Could you check a few things on this model? Use its own coordinates, in mm. Face numbers are marked on the shaded views. A direction names the side the tool comes from. Give positions to 0.01 mm unless a question says otherwise; leave off trailing zeros. Write each loop counter-clockwise with the first axis right and the second up, starting at its lowest first coordinate (ties: lowest second). Pieces come first, ordered by that corner, then holes. Notation, with made-up numbers: (67.25, -16.5) - (111.25, -16.5) arc R29 cw to (111.25, 10.5) - close; hole circle Ø2 at (-29.5, 24). An arc over 180 degrees is marked (long way). Answer as a JSON object with one key per item and string values. Group by question number.
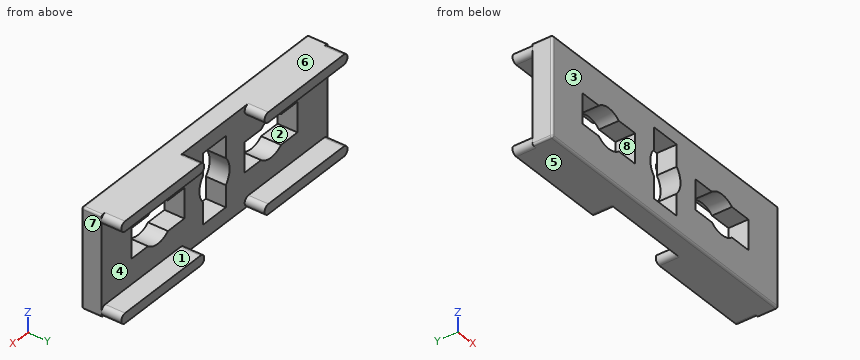
```python
from build123d import *

# Parameters (mm, degrees)
SKETCH_1_W            = 30
SKETCH_1_H            = 10
EXTRUDE_1_DEPTH       = 2
EXTRUDE_2_DEPTH       = 2
MIRROR_2_COPY_1_DEPTH = 2
CUT_EXTRUDE_1_REACH   = 17.937
CUT_EXTRUDE_2_REACH   = 17.937
FILLET_1_R            = 0.2


with BuildPart() as part:
    # 草图1 → 凸台-拉伸1 (new body)
    with BuildSketch(Plane(origin=(0, 0, 0), x_dir=(1, 0, 0), z_dir=(0, 1, 0))):
        Rectangle(SKETCH_1_W, SKETCH_1_H)
    extrude(amount=EXTRUDE_1_DEPTH)

    # 草图2 → 凸台-拉伸2 (add)
    with BuildSketch(Plane(origin=(0, 2, 0), x_dir=(1, 0, 0), z_dir=(0, 1, 0))):
        with BuildLine():
            Line((-14.5, 4), (-4.5, 4))
            ThreePointArc((-4.5, 4), (-4, 4.5), (-4.5, 5))
            Line((-4.5, 5), (-14.5, 5))
            ThreePointArc((-14.5, 5), (-15, 4.5), (-14.5, 4))
        make_face()
    extrude_2 = extrude(amount=EXTRUDE_2_DEPTH)

    # 镜向1: 凸台-拉伸2 across plane
    add(extrude_2.mirror(Plane.XY))

    # 镜向2: 凸台-拉伸2 across plane
    add(extrude_2.mirror(Plane(origin=(0, 0, 0), x_dir=(0, 0, 1), z_dir=(1, 0, 0))))

    # 镜向2 copy 1 sketch → 镜向2 copy 1 (add)
    with BuildSketch(Plane(origin=(0, 2, 0), x_dir=(-1, 0, 0), z_dir=(0, 1, 0))):
        with BuildLine():
            Line((-14.5, 4), (-4.5, 4))
            ThreePointArc((-4.5, 4), (-4, 4.5), (-4.5, 5))
            Line((-4.5, 5), (-14.5, 5))
            ThreePointArc((-14.5, 5), (-15, 4.5), (-14.5, 4))
        make_face()
    extrude(amount=MIRROR_2_COPY_1_DEPTH)

    # 草图3 → 切除-拉伸1 (cut, up to next)
    with BuildSketch(Plane(origin=(0, 2, 0), x_dir=(1, 0, 0), z_dir=(0, 1, 0)), mode=Mode.PRIVATE) as cut_extrude_1_sk1:
        with BuildLine():
            Line((1.5, -3.5), (-1.5, -3.5))
            Line((-1.5, -3.5), (-1.5, -1.322875656))
            ThreePointArc((-1.5, -1.322875656), (-2, 0), (-1.5, 1.322875656))
            Line((-1.5, 1.322875656), (-1.5, 3.5))
            Line((-1.5, 3.5), (1.5, 3.5))
            Line((1.5, 3.5), (1.5, 1.322875656))
            ThreePointArc((1.5, 1.322875656), (2, 0), (1.5, -1.322875656))
            Line((1.5, -1.322875656), (1.5, -3.5))
        make_face()
    cut_extrude_1_tool1 = extrude(cut_extrude_1_sk1.sketch, amount=-CUT_EXTRUDE_1_REACH, mode=Mode.PRIVATE) & part.part
    add(cut_extrude_1_tool1.solids().sort_by_distance((0, 2, 0))[0], mode=Mode.SUBTRACT)

    # 草图4 → 切除-拉伸2 (cut, up to next)
    with BuildSketch(Plane(origin=(0, 2, 0), x_dir=(1, 0, 0), z_dir=(0, 1, 0)), mode=Mode.PRIVATE) as cut_extrude_2_sk1:
        with BuildLine():
            Line((-4, 1.5), (-4, -1.5))
            Line((-4, -1.5), (-6.177124344, -1.5))
            ThreePointArc((-6.177124344, -1.5), (-7.5, -2), (-8.822875656, -1.5))
            Line((-8.822875656, -1.5), (-11, -1.5))
            Line((-11, -1.5), (-11, 1.5))
            Line((-11, 1.5), (-8.822875656, 1.5))
            ThreePointArc((-8.822875656, 1.5), (-7.5, 2), (-6.177124344, 1.5))
            Line((-6.177124344, 1.5), (-4, 1.5))
        make_face()
    cut_extrude_2_tool1 = extrude(cut_extrude_2_sk1.sketch, amount=-CUT_EXTRUDE_2_REACH, mode=Mode.PRIVATE) & part.part
    cut_extrude_2 = cut_extrude_2_tool1.solids().sort_by_distance((-7.5, 2, 0))[0]
    add(cut_extrude_2, mode=Mode.SUBTRACT)

    # 镜向3: 切除-拉伸2 across plane
    add(cut_extrude_2.mirror(Plane(origin=(0, 0, 0), x_dir=(0, 0, 1), z_dir=(1, 0, 0))), mode=Mode.SUBTRACT)

    # 圆角1
    fillet_1_edges = [part.edges().sort_by_distance(p)[0] for p in [
        (0, 0, 5),
        (-15, 1, 5),
        (-15, 0, 0),
        (-15, 1, -5),
        (0, 0, -5),
        (15, 0, 0),
        (15, 1, -5),
        (15, 1, 5),
    ]]
    fillet(fillet_1_edges, radius=FILLET_1_R)


solid = part.part
```
(1) I need wall thicknesses on L1, parallel to X at y = 1.05, z = 0; L2, parallel to Z at x = 9, y = 2.3; L3, parallel to X at y = 1.25, z = -0.5. Which ranges of each line are inside material? Lowest first, please.
(2) If we mould it in two halves opening along X, with no side actions, what happens to the marked faces 6, 7 and 8? For each: +X half, -X half, draft (parallel to the pull), parting line (faces both ways), or undercut.
(3) Will this pin go through, and if not, where does the flat tip stop? P1, Ø3, axis at x = 1, z = 0, coming from the +Y side.
(4) I want a section at A-A, the plane x = 5.25. Please give me the cut outline in (y, z).
(5) I want a section at B-B, the plane y = 2.65. Please give me the cut outline in (x, z), and give its area (3 significant figures).
(6) I want a section at C-C, the plane z = -1. Please give me the cut outline in (x, y).
(7) For the marked faces 1, 2, 3, 4 and 5, which set-ups out of +Z, -Z, +X, -X, +Y, -Y let a thin tool reach every point of the face, with its end or its side?
(8) I want a section at D-D, the plane y = 1.1. State how many separate pieces and enclosed holes the cut face has, and give its area (3 significant figures).
Entries:
{
 "1": {"L1": "-15 to -11, -4 to -2, 2 to 4, 11 to 15", "L2": "-5 to -4, 4 to 5", "L3": "-15 to -11, -4 to -1.94, 1.94 to 4, 11 to 15"},
 "2": {"face 6": "draft", "face 7": "+X half", "face 8": "undercut"},
 "3": {"P1": "y = 2"},
 "4": {"outline": "(0, -4.8) arc R0.2 ccw to (0.2, -5) - (4, -5) - (4, -4) - (2, -4) - (2, -1.5) - (0, -1.5) - close; (0, 1.5) - (2, 1.5) - (2, 4) - (4, 4) - (4, 5) - (0.2, 5) arc R0.2 ccw to (0, 4.8) - close"},
 "5": {"outline": "(-14.5, -5) - (-4.5, -5) arc R0.5 ccw to (-4.5, -4) - (-14.5, -4) arc R0.5 ccw to start; (-14.5, 4) - (-4.5, 4) arc R0.5 ccw to (-4.5, 5) - (-14.5, 5) arc R0.5 ccw to start; (4.5, -5) - (14.5, -5) arc R0.5 ccw to (14.5, -4) - (4.5, -4) arc R0.5 ccw to start; (4.5, 4) - (14.5, 4) arc R0.5 ccw to (14.5, 5) - (4.5, 5) arc R0.5 ccw to start", "area": "43.1 mm^2"},
 "6": {"outline": "(-15, 0.2) arc R0.2 ccw to (-14.8, 0) - (-11, 0) - (-11, 2) - (-15, 2) - close; (-4, 0) - (-1.73, 0) - (-1.73, 2) - (-4, 2) - close; (1.73, 0) - (4, 0) - (4, 2) - (1.73, 2) - close; (11, 0) - (14.8, 0) arc R0.2 ccw to (15, 0.2) - (15, 2) - (11, 2) - close"},
 "7": {"face 1": "+X, -X, +Y", "face 2": "+Y, -Y", "face 3": "+Z, -Z, +X, -X, -Y", "face 4": "+Y", "face 5": "-Z, +X, -X, +Y, -Y"},
 "8": {"separate pieces": "1", "enclosed holes": "3", "area": "232 mm^2"}
}
